Autodesk Inventor part; units mm, degrees
ref_plane "YZ Plane" through (0, 0, 0) normal (1, 0, 0) x (0, 1, 0)
ref_plane "XZ Plane" through (0, 0, 0) normal (0, 1, 0) x (-1, 0, 0)
ref_plane "XY Plane" through (0, 0, 0) normal (0, 0, 1) x (1, 0, 0)
sketch "Sketch1" plane through (0, 0, 0) normal (0, 1, 0) x (-1, 0, 0)
  circle A0 centre (0, 0) radius 50
  dimension "d0" = 100
extrude "Extrusion1" add sketch "Sketch1" along normal blind 2
sketch "Sketch2" plane through (0, 2, 0) normal (0, 1, 0) x (1, 0, 0)
  circle A0 centre (0, 0) radius 49
  dimension "d3" = 98
extrude "Extrusion2" add sketch "Sketch2" along normal blind 2
sketch "Sketch3" plane through (0, 4, 0) normal (0, 1, 0) x (1, 0, 0)
  circle A0 centre (0, 0) radius 50
  dimension "d6" = 100
extrude "Extrusion3" add sketch "Sketch3" along normal blind 2
sketch "Sketch4" plane through (0, 6, 0) normal (0, 1, 0) x (1, 0, 0)
  circle A0 centre (0, 0) radius 10
  dimension "d9" = 20
extrude "Extrusion4" add sketch "Sketch4" along normal blind 20
sketch "Sketch5" plane through (0, 0, 0) normal (0, 0, 1) x (1, 0, 0)
  circle A0 centre (0, 17) radius 1
  point P0 (0, 0)
  dimension "d12" = 2
extrude "Extrusion5" cut sketch "Sketch5" along normal mid plane 25
sketch "Sketch6" plane through (0, 26, 0) normal (0, 1, 0) x (1, 0, 0)
  circle A0 centre (0, 0) radius 2.5
  dimension "d15" = 5
extrude "Extrusion6" cut sketch "Sketch6" against normal blind 20
properties part number "trail 4" material "Polypropylene"
Design review of the part built by this model. Coordinates are the model's own, in mm. A direction names the side the tool comes from. Coordinates: 2 decimals unless noted, no trailing zeros. Order: outer loops, then holes, each group sorted by start corner. A loop starts at its lowest first (then second) coordinate and runs counter-clockwise, first axis right, second up.
Item 1: Take a section at A-A, the plane z = 0. Write out the cut boundary in (x, y), then the cut area to 3 significant figures.
Item 2: For faces 1 (the flat face through (2, 26, 2)), 2 (the cylindrical face through (1.15, 16.14, 2.22)), 3 (the flat face through (37, 4, 33)), list the 3-axis set-ups (+Z, -Z, +X, -X, +Y, -Y) from which the entire face can be reached by the end or side of a thin tool; tool diameter is ignored.
Item 3: For pin 1 Ø8 at (x, z) = (12.5, -39.5) entering from +Y; pin 2 Ø3 at (x, y) = (0, 17) entering from +Z; pin 3 Ø8 at (y, z) = (7, -5.5) entering from +X, all flat-tipped, find the tip position at first contact; note any pin that passes through.
Item 4: For line 1 (Y direction, x = 0, z = 7.75); line 2 (X direction, y = 16, z = 0); line 3 (Y direction, x = 37.5, z = 6), list the stretches that pass through material, from the lowest coordinate up.
Item 5: Take a section at B-B, the plane y = 21.75. Write out the cut boundary in (x, z).
Item 6: Take a section at C-C, the plane x = 25. Write out the cut boundary in (y, z), then the cut area to 3 significant figures.
Item 7: The part is to be moulded in two halves that separate along Y. For faces 4 (the cylindrical face through (26.34, 2.99, 41.32)), 5 (the cylindrical face through (-47.69, 0.99, -15.02)), 6 (the flat face through (0, 6, 0)), say which applies: pulls with the +Y half, pulls with the -Y half, needs draft (parallel to the pull), parting line crosses it, or undercut.
Item 8: Take a section at D-D, the plane z = -33.5. Write out the cut boundary in (x, y), then the cut area to 3 significant figures.
The answers:
1. outline: (-50, 0) - (50, 0) - (50, 2) - (49, 2) - (49, 4) - (50, 4) - (50, 6) - (10, 6) - (10, 26) - (2.5, 26) - (2.5, 6) - (-2.5, 6) - (-2.5, 26) - (-10, 26) - (-10, 6) - (-50, 6) - (-50, 4) - (-49, 4) - (-49, 2) - (-50, 2) - close
1. area: 896 mm2
2. face 1: +Z, -Z, +X, -X, +Y
2. face 2: +Y
2. face 3: none
3. pin 1: stops at y = 6
3. pin 2: stops at z = 10
3. pin 3: stops at x = 49.97
4. line 1: y = 0 to 16, 18 to 26
4. line 2: x = -10 to -2.5, 2.5 to 10
4. line 3: y = 0 to 6
5. outline: circle Ø20 at (0, 0); hole circle Ø5 at (0, 0)
6. outline: (0, -43.3) - (2, -43.3) - (2, -42.14) - (4, -42.14) - (4, -43.3) - (6, -43.3) - (6, 43.3) - (4, 43.3) - (4, 42.14) - (2, 42.14) - (2, 43.3) - (0, 43.3) - close
6. area: 515 mm2
7. face 4: undercut
7. face 5: needs draft
7. face 6: pulls with the +Y half
8. outline: (-37.12, 0) - (37.12, 0) - (37.12, 2) - (35.76, 2) - (35.76, 4) - (37.12, 4) - (37.12, 6) - (-37.12, 6) - (-37.12, 4) - (-35.76, 4) - (-35.76, 2) - (-37.12, 2) - close
8. area: 440 mm2
